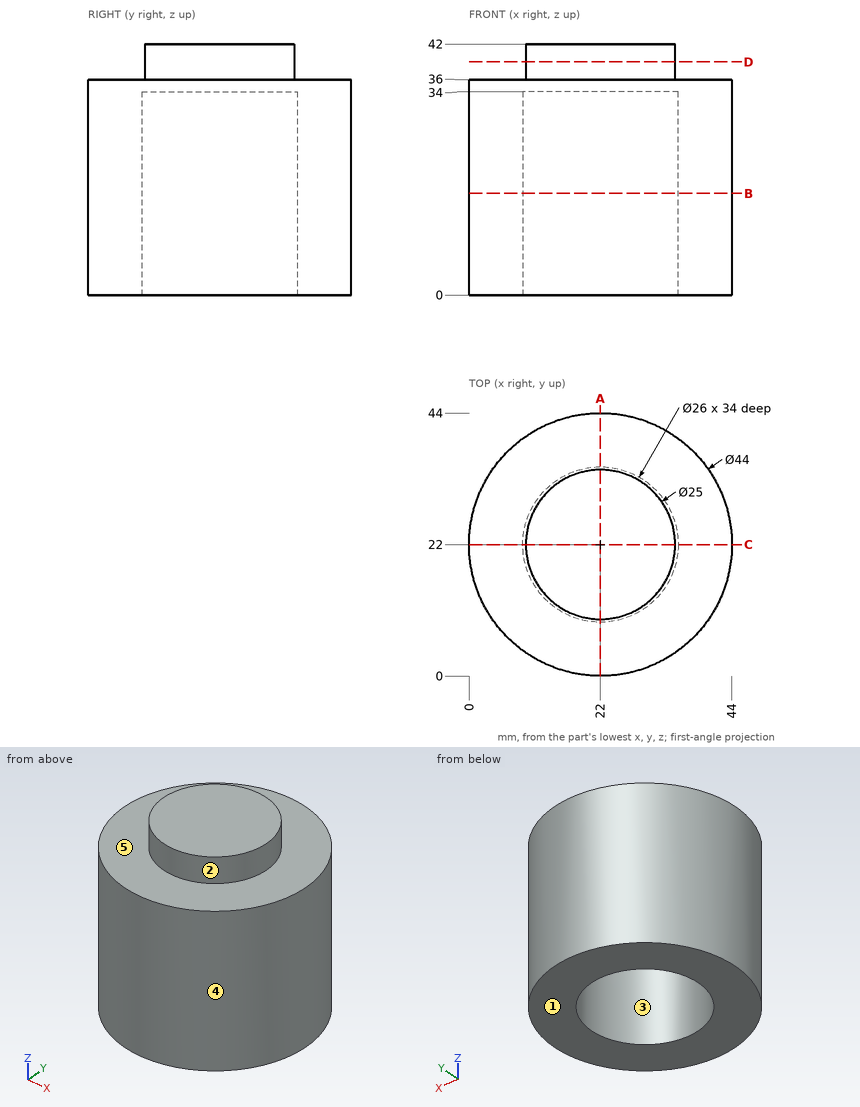
Answer from the drawing. Dimensions are ordinates in mm from the lowest x, y and z of the part. A direction names the side the tool comes from. Round coordinates to 2 decimals unless told otherwise and drop trailing zeros. Write each loop counter-clockwise with the first axis right and the second up, starting at its lowest first coordinate (ties: lowest second). Pieces come first, ordered by that corner, then holes. Notation, with made-up numbers: (81, -24.5) - (92, -24.5) arc R28 ccw to (92, 13.5) - close; hole circle Ø4 at (32, -37.75). An arc over 180 degrees is marked (long way). Use a Markdown table: item, result.
(1) The part is cut by section B-B (z = 17). Write down the section's boundary in (x, y), then the cut area to 3 significant figures.
Reported:
| item | result |
|---|---|
| outline | circle Ø44 at (22, 22); hole circle Ø26 at (22, 22) |
| area | 990 mm2 |
(2) The part is cut by section A-A (x = 22). Write down the section's boundary in (y, z), then the cut area to 3 significant figures.
Reported:
| item | result |
|---|---|
| outline | (0, 0) - (9, 0) - (9, 34) - (35, 34) - (35, 0) - (44, 0) - (44, 36) - (34.5, 36) - (34.5, 42) - (9.5, 42) - (9.5, 36) - (0, 36) - close |
| area | 850 mm2 |
(3) The mould has two halves that part along X. Classify the marked faces 3, 4 and 5: released by +X, released by -X, zero draft, split by the parting line, or undercut.
Reported:
| item | result |
|---|---|
| face 3 | undercut |
| face 4 | split by the parting line |
| face 5 | zero draft |
(4) The part is cut by section D-D (z = 39). Write down the section's boundary in (x, y), then the cut area to 3 significant figures.
Reported:
| item | result |
|---|---|
| outline | circle Ø25 at (22, 22) |
| area | 491 mm2 |
(5) Each of these flat-tipped pins is pushed along its axis until it touches: pin 1 Ø8 at (x, z) = (23.5, 30.5) entering from -Y; pin 2 Ø4 at (y, z) = (36, 4.5) entering from +X; pin 3 Ø3 at (y, z) = (28, 8) entering from +X; pin 4 Ø1 at (x, y) = (5.5, 25) entering from -Z. Where does it stop, or does it pass through?
Reported:
| item | result |
|---|---|
| pin 1 | y = 0 |
| pin 2 | x = 40.44 |
| pin 3 | x = 43.53 |
| pin 4 | z = 0 |
(6) Straight lines are drawn through the part: line 1 along X through (y, z) = (22, 12); line 2 along Y through (x, z) = (15.5, 17). For each, find the intervals that lie inside material, in ascending order. Write a range as [from, to].
Reported:
| item | result |
|---|---|
| line 1 | [0, 9], [35, 44] |
| line 2 | [0.98, 10.74], [33.26, 43.02] |
(7) Which of the six approach directions +Z, -Z, +X, -X, +Y, -Y give full straight-line access (tool end or side, diameter ignored) to the marked faces 1 and 2?
Reported:
| item | result |
|---|---|
| face 1 | -Z, +X, -X, +Y, -Y |
| face 2 | +Z |
